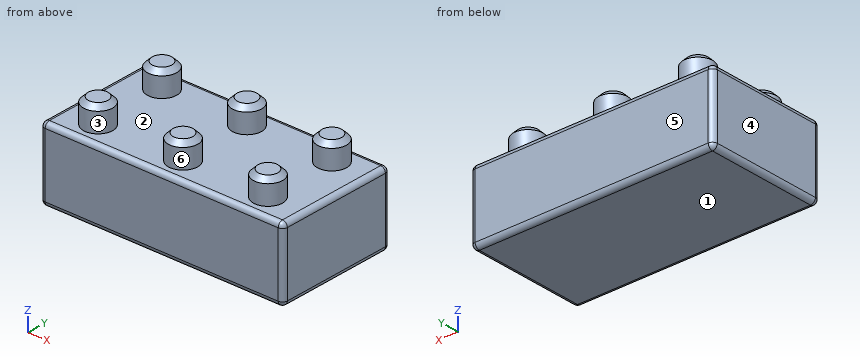
```python
from build123d import *

# Parameters (mm, degrees)
F0_W      = 100
F0_H      = 50
F1_DEPTH  = 30
F2_R      = 6
F3_DEPTH  = 10
F4_R      = 2
F5_SIZE   = 2
F3_FACE_R = 4
F6_DEPTH  = 5


with BuildPart() as f1:
    # F0 (on Top) → F1 (new body)
    with BuildSketch(Plane.XY):
        Rectangle(F0_W, F0_H)
    extrude(amount=F1_DEPTH)

    # F2 (on face) → F3 (join)
    with BuildSketch(Plane.XY.offset(30)):
        with Locations((35, 15)):
            Circle(F2_R)
        with Locations((35, -15)):
            Circle(F2_R)
        with Locations((0, -15)):
            Circle(F2_R)
        with Locations((0, 15)):
            Circle(F2_R)
        with Locations((-35, 15)):
            Circle(F2_R)
        with Locations((-35, -15)):
            Circle(F2_R)
    extrude(amount=F3_DEPTH)

    # F4
    f4_edges = [f1.edges().sort_by_distance(p)[0] for p in [
        (50, 0, 30),
        (0, -25, 30),
        (0, 25, 30),
        (-50, 0, 30),
        (50, -25, 15),
        (50, 25, 15),
        (50, 0, 0),
        (-50, -25, 15),
        (0, -25, 0),
        (-50, 25, 15),
        (0, 25, 0),
        (-50, 0, 0),
    ]]
    fillet(f4_edges, radius=F4_R)

    # F5
    f5_edges = [f1.edges().sort_by_distance(p)[0] for p in [
        (-41, 15, 40),
        (-41, -15, 40),
        (-6, -15, 40),
        (-6, 15, 40),
        (29, 15, 40),
        (29, -15, 40),
    ]]
    chamfer(f5_edges, length=F5_SIZE)

    # F3_face (on face) → F6 (join)
    with BuildSketch(Plane(origin=(-35, -15, 40), x_dir=(1, 0, 0), z_dir=(0, 0, 1))):
        Circle(F3_FACE_R)
    extrude(amount=-F6_DEPTH)


solid = f1.part
```
The model under review builds one solid part; all positions refer to its coordinate system, in mm. Face numbers are marked on the shaded views. A direction names the side the tool comes from. Round coordinates to 2 decimals unless told otherwise and drop trailing zeros. Order: outer loops, then holes, each group sorted by start corner. A loop starts at its lowest first (then second) coordinate and runs counter-clockwise, first axis right, second up. Notation, with made-up numbers: (57.25, 54.25) -> (79.25, 54.25) arc R3 ccw to (79.25, 59.25) -> close; hole circle Ø3 at (85, 13.25). An arc over 180 degrees is marked (long way). Use a Markdown table: item, result.
Q1. We need section D-D on y = -15. Write out the cut boundary in (x, z).
Values:
| item | result |
|---|---|
| outline | (-50, 2) arc R2 ccw to (-48, 0) -> (48, 0) arc R2 ccw to (50, 2) -> (50, 28) arc R2 ccw to (48, 30) -> (41, 30) -> (41, 38) -> (39, 40) -> (31, 40) -> (29, 38) -> (29, 30) -> (6, 30) -> (6, 38) -> (4, 40) -> (-4, 40) -> (-6, 38) -> (-6, 30) -> (-29, 30) -> (-29, 38) -> (-31, 40) -> (-39, 40) -> (-41, 38) -> (-41, 30) -> (-48, 30) arc R2 ccw to (-50, 28) -> close |
Q2. Clearance check with a flat-ended pin moving along its axis: P1, Ø4, axis at x = -21.5, y = -11.5, coming from the +Z side. State where the tip first meets the part, or that it passes through.
Values:
| item | result |
|---|---|
| P1 | stops at z = 30 |
Q3. Tool access review of the marked faces 1 and 2: name each direction out of +Z, -Z, +X, -X, +Y, -Y from which nothing blocks a thin tool from reaching the whole face with its end or side.
Values:
| item | result |
|---|---|
| face 1 | -Z, +X, -X, +Y, -Y |
| face 2 | +Z |
Q4. For line 1 (Z direction, x = -18, y = -21); line 2 (X direction, y = 16.5, z = 31.5); line 3 (Y direction, x = 39, z = 31.5), list the stretches that pass through material, from the lowest coordinate up.
Values:
| item | result |
|---|---|
| line 1 | z = 0 to 30 |
| line 2 | x = -40.81 to -29.19, -5.81 to 5.81, 29.19 to 40.81 |
| line 3 | y = -19.47 to -10.53, 10.53 to 19.47 |
Q5. We need section B-B on x = 35. Write out the cut boundary in (y, z).
Values:
| item | result |
|---|---|
| outline | (-25, 2) arc R2 ccw to (-23, 0) -> (23, 0) arc R2 ccw to (25, 2) -> (25, 28) arc R2 ccw to (23, 30) -> (21, 30) -> (21, 38) -> (19, 40) -> (11, 40) -> (9, 38) -> (9, 30) -> (-9, 30) -> (-9, 38) -> (-11, 40) -> (-19, 40) -> (-21, 38) -> (-21, 30) -> (-23, 30) arc R2 ccw to (-25, 28) -> close |
Q6. Mouldability with a two-part tool opening along Y and no side actions: class the marked faces 3, 4, 5 and 6 as +Y half, -Y half, draft (parallel to the pull), parting line (faces both ways), or undercut.
Values:
| item | result |
|---|---|
| face 3 | undercut |
| face 4 | draft |
| face 5 | +Y half |
| face 6 | undercut |
Q7. We need section A-A on z = 36.5. Write out the cut boundary in (x, y), then the cut area to 3 significant figures.
Values:
| item | result |
|---|---|
| outline | circle Ø12 at (-35, -15); circle Ø12 at (-35, 15); circle Ø12 at (0, -15); circle Ø12 at (0, 15); circle Ø12 at (35, -15); circle Ø12 at (35, 15) |
| area | 679 mm^2 |
Q8. We need section C-C on y = -7. Write out the cut boundary in (x, z).
Values:
| item | result |
|---|---|
| outline | (-50, 2) arc R2 ccw to (-48, 0) -> (48, 0) arc R2 ccw to (50, 2) -> (50, 28) arc R2 ccw to (48, 30) -> (-48, 30) arc R2 ccw to (-50, 28) -> close |
